Here's the drawing with two shaded views (mm, measured from the low corner). I have some questions. A direction names the side the tool comes from. Round coordinates to 2 decimals unless told otherwise and drop trailing zeros. Write each loop counter-clockwise with the first axis right and the second up, starting at its lowest first coordinate (ties: lowest second). Pieces come first, ordered by that corner, then holes. Notation, with made-up numbers: M 33,43.25 L 42,43.25 A23 ccw 42,63.25 Z; hole C 7.25,0 d5. An arc over 180 degrees is marked long. Answer as a JSON object with one key per item and string values. Group by question number.
1) Suppose I cut it at D-D, the plane x = 5. Write out the boundary of the cut face in (y, z), and give its area (3 significant figures).
2) Please list where these lines run through material, in increasing order: L1, parallel to X at y = 1.55, z = 2.54; L2, parallel to Z at x = 2.54, y = 0.85; L3, parallel to X at y = 4, z = 10. Write a range as [from, to].
3) Suppose I cut it at A-A, the plane y = 2.5. Write out the boundary of the cut face in (x, z), and give its area (3 significant figures).
4) Suppose I cut it at C-C, the plane z = 8.5. Write out the boundary of the cut face in (x, y), and give its area (3 significant figures).
5) Suppose I cut it at B-B, the plane y = 1. Write out the boundary of the cut face in (x, z).
6) If we mould it in two halves opening along X, with no side actions, what happens to the marked faces 4, 5 and 6? For each: +X half, -X half, draft (parallel to the pull), parting line (faces both ways), or undercut.
7) I'm going to push flat-ended pins straight in: pin 1 Ø3 at (x, z) = (22.5, 10.5) entering from +Y; pin 2 Ø1.5 at (x, y) = (22, 4) entering from -Z; pin 3 Ø2 at (x, y) = (20, 4) entering from +Z. Where does each tip first touch, or does it pass through?
8) On a 3-axis mill with a long thin cutter (end or side, diameter ignored), from which of +Z, -Z, +X, -X, +Y, -Y can I reach the whole of each face in a straight line? I mean the marked faces 1, 2 and 3. Say none if no direction works.
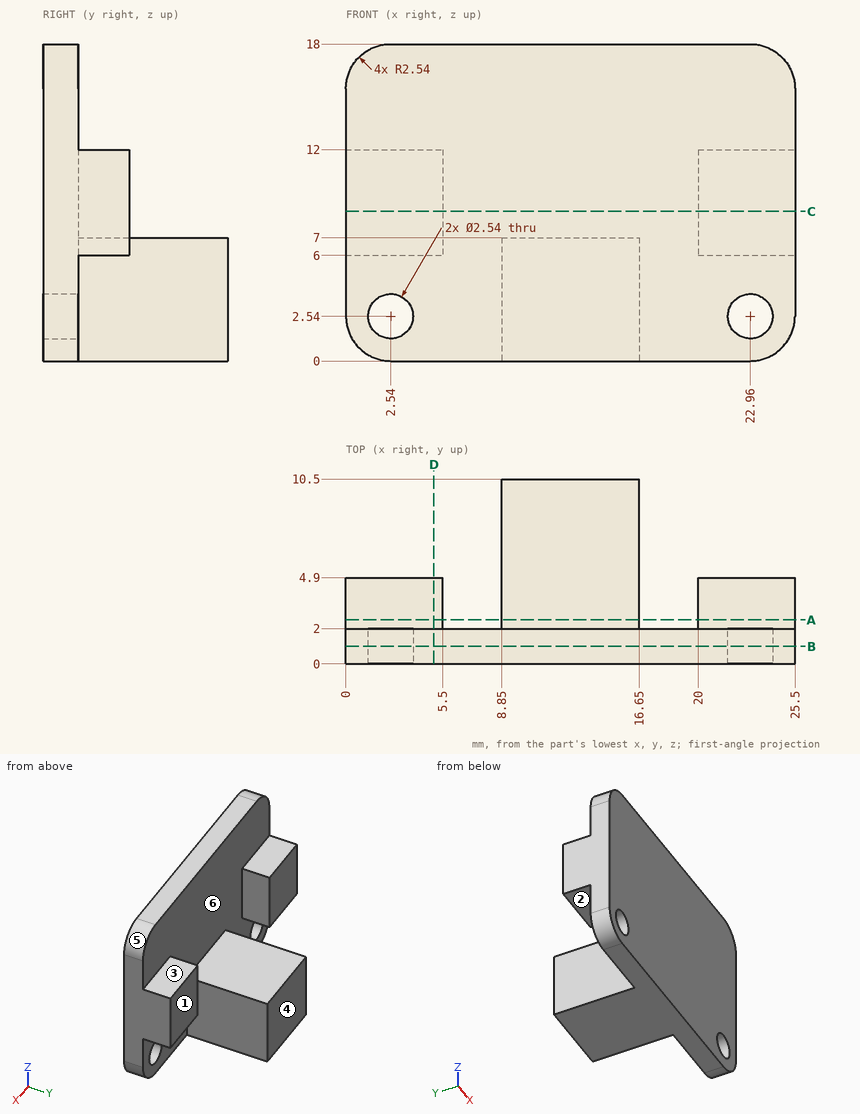
Results:
{
 "1": {"outline": "M 0,0 L 2,0 L 2,6 L 4.9,6 L 4.9,12 L 2,12 L 2,18 L 0,18 Z", "area": "53.4 mm^2"},
 "2": {"L1": "[0, 1.27], [3.81, 21.69], [24.23, 25.5]", "L2": "[0, 1.27], [3.81, 18]", "L3": "[0, 5.5], [20, 25.5]"},
 "3": {"outline": "M 0,6 L 5.5,6 L 5.5,12 L 0,12 Z; M 8.85,0 L 16.65,0 L 16.65,7 L 8.85,7 Z; M 20,6 L 25.5,6 L 25.5,12 L 20,12 Z", "area": "121 mm^2"},
 "4": {"outline": "M 0,0 L 25.5,0 L 25.5,4.9 L 20,4.9 L 20,2 L 5.5,2 L 5.5,4.9 L 0,4.9 Z", "area": "82.9 mm^2"},
 "5": {"outline": "M 0,2.54 A2.54 ccw 2.54,0 L 22.96,0 A2.54 ccw 25.5,2.54 L 25.5,15.46 A2.54 ccw 22.96,18 L 2.54,18 A2.54 ccw 0,15.46 Z; hole C 2.54,2.54 d2.54; hole C 22.96,2.54 d2.54"},
 "6": {"face 4": "draft", "face 5": "+X half", "face 6": "undercut"},
 "7": {"pin 1": "y = 4.9", "pin 2": "z = 6", "pin 3": "z = 12"},
 "8": {"face 1": "+Z, -Z, +X, +Y", "face 2": "-Z, -X, +Y", "face 3": "+Z, +X, -X, +Y"}
}
